Model file for the job. Use its own axes, mm. Round coordinates to 2 decimals unless told otherwise and drop trailing zeros. Order: outer loops, then holes, each group sorted by start corner. A loop starts at its lowest first (then second) coordinate and runs counter-clockwise, first axis right, second up. Notation, with made-up numbers: (54.5, 50.5) - (86.5, 50.5) arc R20 cw to (86.5, 89.5) - close; hole circle Ø1 at (-31, -18). An arc over 180 degrees is marked (long way). Use one line per item in the form item = value.
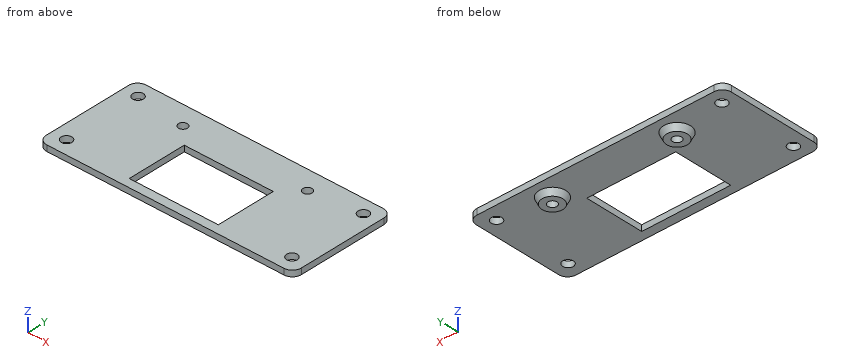
from build123d import *

# Parameters (mm, degrees)
CYLINDER052_R       = 1.5
CYLINDER052_DEPTH   = 20
ARRAY001023_X_COUNT = 2
ARRAY001023_X_PITCH = 42
CYLINDER056_R       = 1.8
CYLINDER056_DEPTH   = 12
ARRAY001028_X_COUNT = 2
ARRAY001028_X_PITCH = 76
ARRAY001028_Y_COUNT = 2
ARRAY001028_Y_PITCH = 26
BOX024_W            = 30
BOX024_H            = 20
BOX024_DEPTH        = 10
BOX023_W            = 86
BOX023_H            = 36
BOX023_DEPTH        = 2
FILLET012_R         = 3
ARRAY001027_X_COUNT = 2
ARRAY001027_X_PITCH = 42


with BuildPart() as obj1:
    # Cylinder052 → Cylinder052 (new body)
    with BuildSketch(Plane(origin=(22, 29, -5), x_dir=(1, 0, 0), z_dir=(0, 0, 1))):
        Circle(CYLINDER052_R)
    extrude(amount=CYLINDER052_DEPTH)

    # Array001023 X: obj1 ×2


with BuildPart() as obj1_1:
    add(obj1.part)
    with Locations(*[(i * ARRAY001023_X_PITCH, 0, 0) for i in range(1, ARRAY001023_X_COUNT)]):
        add(obj1.part)


with BuildPart() as obj2:
    # Cylinder056 → Cylinder056 (new body)
    with BuildSketch(Plane(origin=(5, 5, 0), x_dir=(1, 0, 0), z_dir=(0, 0, 1))):
        Circle(CYLINDER056_R)
    extrude(amount=CYLINDER056_DEPTH)

    # Array001028 X: obj2_2


with BuildPart() as obj2_1:
    add(obj2.part)
    with Locations(*[(i * ARRAY001028_X_PITCH, 0, 0) for i in range(1, ARRAY001028_X_COUNT)]):
        add(obj2.part)

    # Array001028 Y: obj2_2


with BuildPart() as obj2_2:
    add(obj2_1.part)
    with Locations(*[(0, i * ARRAY001028_Y_PITCH, 0) for i in range(1, ARRAY001028_Y_COUNT)]):
        add(obj2_1.part)


with BuildPart() as obj3:
    # Box024 → Box024 (new body)
    with BuildSketch(Plane(origin=(28, 3, -5), x_dir=(1, 0, 0), z_dir=(0, 0, 1))):
        with Locations((15, 10)):
            Rectangle(BOX024_W, BOX024_H)
    extrude(amount=BOX024_DEPTH)

    # Fusion034: union obj1, obj2
    add(obj1_1.part)
    add(obj2_2.part)


with BuildPart() as obj4:
    # Box023 → Box023 (new body)
    with BuildSketch(Plane.XY):
        with Locations((43, 18)):
            Rectangle(BOX023_W, BOX023_H)
    extrude(amount=BOX023_DEPTH)

    # Fillet012
    fillet012_edges = [obj4.edges().sort_by_distance(p)[0] for p in [
        (0, 0, 1),
        (0, 36, 1),
        (86, 0, 1),
        (86, 36, 1),
    ]]
    fillet(fillet012_edges, radius=FILLET012_R)


with BuildPart() as obj5:
    # Cone003 → Cone003 (revolve)
    with BuildSketch(Plane(origin=(22, 29, -2), x_dir=(1, 0, 0), z_dir=(0, -1, 0))):
        Polygon((0, 0), (3.5, 0), (5, 3), (0, 3), align=None)
    revolve(axis=Axis((22, 29, -2), (0, 0, 1)))

    # Array001027 X: obj5_2


with BuildPart() as obj5_1:
    add(obj5.part)
    with Locations(*[(i * ARRAY001027_X_PITCH, 0, 0) for i in range(1, ARRAY001027_X_COUNT)]):
        add(obj5.part)

    # Fusion038: union obj4
    add(obj4.part)

    # Cut021: cut obj3
    add(obj3.part, mode=Mode.SUBTRACT)


with BuildPart() as obj5_2:
    # Cut021 placement: moved
    add(obj5_1.part.moved(Location((0, 0, 12))))


solid = obj5_2.part
(1) Pin check, flat tips, straight feed: pin 1 (2 mm diameter, centred on x = 5, y = 31, fed in from +Z); pin 2 (6 mm diameter, centred on x = 5, y = 5, fed in from -Z). Stop position of each tip, or through.
Report:
pin_1 = through
pin_2 = 12
(2) Slice it at B-B on x = 49. Give the cut face in (y, z).
Report:
outline = (0, 12) - (3, 12) - (3, 14) - (0, 14) - close; (23, 12) - (36, 12) - (36, 14) - (23, 14) - close
(3) Slice it at C-C on y = 8.5. Give the cut face in (x, z).
Report:
outline = (0, 12) - (28, 12) - (28, 14) - (0, 14) - close; (58, 12) - (86, 12) - (86, 14) - (58, 14) - close
(4) Slice it at D-D on x = 81. Give the cut face in (y, z).
Report:
outline = (0, 12) - (3.2, 12) - (3.2, 14) - (0, 14) - close; (6.8, 12) - (29.2, 12) - (29.2, 14) - (6.8, 14) - close; (32.8, 12) - (36, 12) - (36, 14) - (32.8, 14) - close
(5) Probe probe 1 along X at (y, z) = (31, 13); probe 2 along Y at (x, z) = (81, 13.1); probe 3 along X at (y, z) = (5, 12.9). List the from-to ranges inside material, lowest first. Write a range as [from, to].
Report:
probe_1 = [0, 3.2], [6.8, 79.2], [82.8, 86]
probe_2 = [0, 3.2], [6.8, 29.2], [32.8, 36]
probe_3 = [0, 3.2], [6.8, 28], [58, 79.2], [82.8, 86]
(6) Slice it at A-A on z = 12.95. Give the cut face in (x, y), then the cut area to 3 significant figures.
Report:
outline = (0, 3) arc R3 ccw to (3, 0) - (83, 0) arc R3 ccw to (86, 3) - (86, 33) arc R3 ccw to (83, 36) - (3, 36) arc R3 ccw to (0, 33) - close; hole circle Ø3.6 at (5, 5); hole circle Ø3.6 at (5, 31); hole circle Ø3 at (22, 29); hole (28, 3) - (58, 3) - (58, 23) - (28, 23) - close; hole circle Ø3 at (64, 29); hole circle Ø3.6 at (81, 5); hole circle Ø3.6 at (81, 31)
area = 2,430 mm2
